Source: CAD feature listing. Evaluate the final solid. Frame: model axes, mm. Face numbers are marked on the shaded views. Round coordinates to 2 decimals unless told otherwise and drop trailing zeros. Answer in a Markdown table with one row per item.
from build123d import *

# Parameters (mm, degrees)
SKETCH1_W           = 255
SKETCH1_H           = 110
SKETCH1_R           = 1.5
BOSS_EXTRUDE1_DEPTH = 3


with BuildPart() as part:
    # Sketch1 → Boss-Extrude1 (new body)
    with BuildSketch(Plane.XY):
        with Locations((-13.136363636, -6.318181818)):
            Rectangle(SKETCH1_W, SKETCH1_H)
        with Locations((-125.636363636, -49.318181818)):
            Circle(SKETCH1_R, mode=Mode.SUBTRACT)
        with Locations((-133.636363636, 32.681818182)):
            Circle(SKETCH1_R, mode=Mode.SUBTRACT)
        with Locations((99.363636364, -47.318181818)):
            Circle(SKETCH1_R, mode=Mode.SUBTRACT)
        with Locations((99.363636364, 35.681818182)):
            Circle(SKETCH1_R, mode=Mode.SUBTRACT)
        with Locations((-97.369202936, 23.681818182)):
            Circle(SKETCH1_R, mode=Mode.SUBTRACT)
        with Locations((-97.369202936, -36.318181818)):
            Circle(SKETCH1_R, mode=Mode.SUBTRACT)
        with Locations(Location((71.096475664, -36.318181818, 0), (0, 0, 180))):
            Circle(SKETCH1_R, mode=Mode.SUBTRACT)
        with Locations(Location((71.096475664, 23.681818182, 0), (0, 0, 180))):
            Circle(SKETCH1_R, mode=Mode.SUBTRACT)
        with Locations((-13.136363636, -6.318181818)):
            Circle(SKETCH1_R, mode=Mode.SUBTRACT)
    extrude(amount=BOSS_EXTRUDE1_DEPTH)


solid = part.part
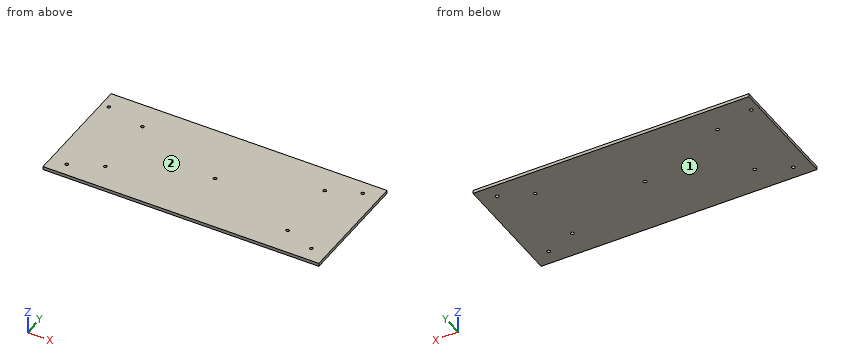
Q1. Material intervals for probe 1 along X at (y, z) = (33, 2.5); probe 2 along Y at (x, z) = (-14.5, 1.5); probe 3 along X at (y, z) = (32, 2.4), sorted ascending.
Solutions:
| item | result |
|---|---|
| probe 1 | x = -140.64 to -135.1, -132.17 to 114.36 |
| probe 2 | y = -61.32 to -6.94, -5.69 to 48.68 |
| probe 3 | x = -140.64 to -134.97, -132.3 to 114.36 |
Q2. Contact query for a flat-ended pin moving along its axis: pin 1 Ø1.8 at (x, y) = (-97.37, 23.68) entering from -Z. Output: stop coordinate, or through.
Solutions:
| item | result |
|---|---|
| pin 1 | passes through |
Q3. Pull-direction query (Z, two-part tool) for the marked faces 1 and 2; classes: pulls with the +Z half, pulls with the -Z half, needs draft (parallel to the pull), parting line crosses it, or undercut.
Solutions:
| item | result |
|---|---|
| face 1 | pulls with the -Z half |
| face 2 | pulls with the +Z half |
